Geometry: final body of the model. Coordinates: model frame, mm. A direction names the side the tool comes from. Give positions to 0.01 mm unless a question says otherwise; leave off trailing zeros. Loops run counter-clockwise (first coordinate to the right, second up) from the corner with the lowest first, then second, coordinate; pieces in that order, holes last. Notation, with made-up numbers: (89.25, -37) -> (101.25, -37) arc R31 cw to (101.25, 1) -> close; hole circle Ø11 at (78, -13). An arc over 180 degrees is marked (long way). One line per question, with ' | ' between items. Start each with the question number.
Item 1: Set-up query: faces 4 (the flat face through (6.783, 213, 2)), 5 (the flat face through (-4, 213, -10.401)). Return all of +Z, -Z, +X, -X, +Y, -Y with unobstructed straight access to the full face (end or side cutting, diameter ignored); none if empty.
Item 2: Section B-B on y = 200. Return loops of the section in (x, z).
Item 3: Pin query (flat end, axial travel): P1, Ø7.5, axis at y = 107.95, z = -4.051, coming from the -X side. Return the tip coordinate at first contact, or that it passes through.
Item 4: Mould query, pull axis X, two halves, no side actions, for faces 1 (the flat face through (8.37, 213, 2)), 2 (the flat face through (7, 0, 2)), 3 (the flat face through (-4, 213, -8.814)). Classes: released by +X, released by -X, zero draft, split by the parting line, or undercut.
Item 5: Section A-A on x = 0. Return loops of the section in (y, z).
Item 6: Material intervals for line 1 along Z through (x, y) = (0, 283.5); line 2 along X through (y, z) = (342.5, 4.25); line 3 along Z through (x, y) = (-15.85, 95.25), sorted ascending. Write a range as [from, to].
Autodesk Inventor part; units mm, degrees
ref_plane "YZ Plane" through (0, 0, 0) normal (1, 0, 0) x (0, 1, 0)
ref_plane "XZ Plane" through (0, 0, 0) normal (0, 1, 0) x (-1, 0, 0)
ref_plane "XY Plane" through (0, 0, 0) normal (0, 0, 1) x (1, 0, 0)
sketch "Sketch1" plane through (0, 0, 0) normal (0, 1, 0) x (-1, 0, 0)
  line L0 (17.0295, 14.999) -> (-8.3705, 14.999)
  line L1 (-8.3705, 14.999) -> (-8.3705, -10.401)
  line L2 (-8.3705, -10.401) -> (17.0295, -10.401)
  line L3 (17.0295, -10.401) -> (17.0295, 14.999)
  line L4 (15.442, -8.8135) -> (-6.783, -8.8135)
  line L5 (-6.783, -8.8135) -> (-6.783, 13.4115)
  line L6 (-6.783, 13.4115) -> (15.442, 13.4115)
  line L7 (15.442, 13.4115) -> (15.442, -8.8135)
  point P0 (0, 0)
  dimension "d0" = 25.4
  dimension "d1" = 25.4
  dimension "d4" = 1.5875
  dimension "d5" = 1.5875
  dimension "d6" = 1.5875
  dimension "d7" = 1.5875
extrude "Extrusion2" add sketch "Sketch1" along normal blind 431.8
sketch "Sketch3" plane through (8.3705, 0, 14.999) normal (1, 0, 0) x (0, 0, -1)
  line L0 (25.4, 0) -> (25.4, 431.8)
  line L1 (0, 431.8) -> (25.4, 431.8)
  line L2 (0, 0) -> (25.4, 0)
  point P0 (14.999, 0)
  point P1 (19.05, 349.25)
  point P2 (19.05, 82.55)
  dimension "d19" = 6.35
  dimension "d20" = 82.55
  dimension "d21" = 6.35
  dimension "d22" = 82.55
hole "Hole2" at (8.3705, 349.25, -4.051) at (8.3705, 82.55, -4.051) direction (-1, 0, 0) diameter 4.7625 depth 25.4 tip angle 118.188
sketch "Sketch4" plane through (8.3705, 0, 14.999) normal (1, 0, 0) x (0, 0, -1)
  line L0 (25.4, 0) -> (25.4, 431.8)
  circle A0 centre (19.05, 82.55) radius 2.3813
  line L1 (0, 0) -> (0, 431.8)
  circle A1 centre (19.05, 349.25) radius 2.3813
  point P0 (14.999, 0)
  point P1 (19.05, 107.95)
  point P2 (6.35, 69.85)
  point P3 (6.35, 95.25)
  point P4 (19.05, 323.85)
  point P5 (6.35, 361.95)
  point P6 (6.35, 336.55)
  dimension "d30" = 6.35
  dimension "d31" = 25.4
  dimension "d32" = 6.35
  dimension "d33" = 6.35
  dimension "d34" = 25.4
  dimension "d36" = 6.35
  dimension "d37" = 25.4
  dimension "d38" = 6.35
  dimension "d39" = 6.35
  dimension "d40" = 25.4
  dimension "d49" = 12.7
  dimension "d50" = 12.7
hole "Hole3" at (8.3705, 107.95, -4.051) at (8.3705, 69.85, 8.649) at (8.3705, 95.25, 8.649) at (8.3705, 323.85, -4.051) at (8.3705, 361.95, 8.649) at (8.3705, 336.55, 8.649) direction (-1, 0, 0) diameter 4.7625 depth 25.4 tip angle 118.188
equation "\"d0\" = ElvBeamWidth"
equation "\"d1\" = ElvBeamWidth"
equation "\"d4\" = ElvWallWidth"
equation "\"d5\" = ElvWallWidth"
equation "\"d6\" = ElvWallWidth"
equation "\"d7\" = ElvWallWidth"
equation "\"d8\" = ElvEndEffectLength"
equation "\"ElvMiddleBeamLength\" = 990.6"
equation "\"ElvWallWidth\" = 1.5875"
equation "\"ElvFrontBeamLength\" = 990.6"
equation "\"ElvEndEffectLength\" = 431.8"
equation "\"ElvCrossBeamLength\" = 304.8"
equation "\"ElvBeamWidth\" = 25.4"
equation "\"ElvFrontBeamLength_1\" = 1066.8"
equation "\"ElvFixedBeamLength\" = 990.6"
equation "\"ElvDelHeight\" = 101.6"
equation "\"ElvDelFrontTabLength\" = 6.35"
equation "\"ElvDelWidth\" = 18.542"
equation "\"ElvDelDepth\" = 6.35"
equation "\"ElvTopBeamLength\" = 457.2"
equation "\"ElvHoleFromFixed\" = 50.8"
equation "\"ElvHoleFromMid\" = 38.1"
equation "\"ElvHoleFromFront\" = 25.4"
equation "\"ElvHoleFromBottom\" = 38.1"
equation "\"ElvRivetPlateLength\" = 76.2"
equation "\"ElvDelMiddleTabLength\" = 6.35"
properties part number "ElvEndEffectBeam" material "Aluminum 6061"
Result sheet:
1) face 4: +Y, -Y | face 5: -Z, +X, -X, +Y, -Y
2) outline: (-17.03, -10.4) -> (8.37, -10.4) -> (8.37, 15) -> (-17.03, 15) -> close; hole (-15.44, -8.81) -> (6.78, -8.81) -> (6.78, 13.41) -> (-15.44, 13.41) -> close
3) P1: stops at x = -17.03
4) face 1: released by +X | face 2: zero draft | face 3: undercut
5) outline: (0, -10.4) -> (431.8, -10.4) -> (431.8, -8.81) -> (0, -8.81) -> close; (0, 13.41) -> (431.8, 13.41) -> (431.8, 15) -> (0, 15) -> close
6) line 1: z = [-10.4, -8.81], [13.41, 15] | line 2: x = [-17.03, -15.44], [6.78, 8.37] | line 3: z = [-10.4, 6.27], [11.03, 15]
